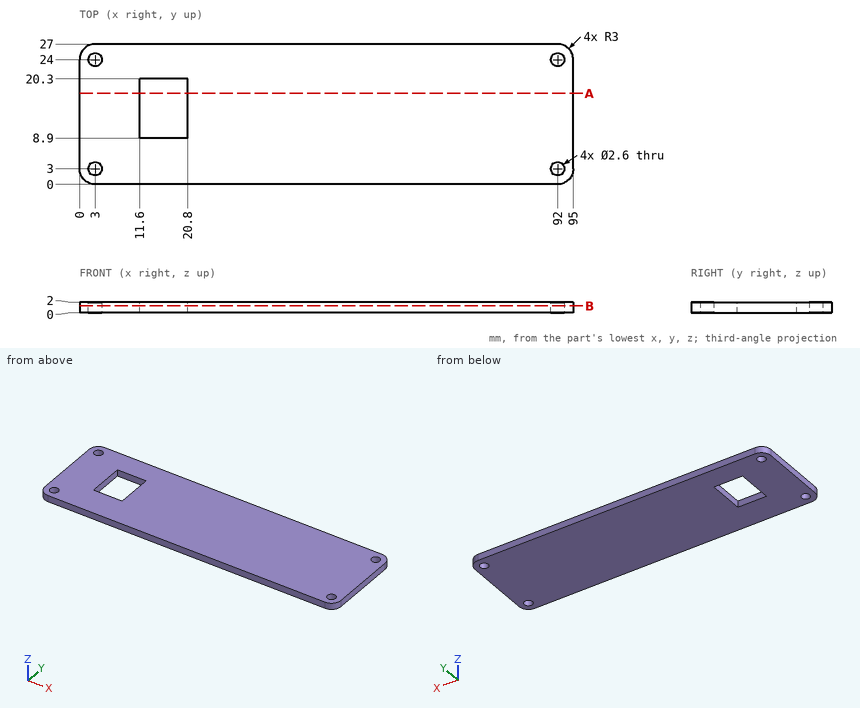
The figure shows three views and two pictorial views of one solid part (mm, origin at its lowest corner). Answer the questions. Coordinates: 2 decimals unless noted, no trailing zeros. Write each loop counter-clockwise with the first axis right and the second up, starting at its lowest first coordinate (ties: lowest second). Pieces come first, ordered by that corner, then holes. Notation, with made-up numbers: (3, 30) -> (28, 30) arc R30 cw to (28, 65) -> close; hole circle Ø9 at (53, 61). An arc over 180 degrees is marked (long way). Answer as a JSON object with one key per item and string values.
Q1. Consider line 1 (Y direction, x = 3, z = 1.15); line 2 (X direction, y = 10.75, z = 1.35); line 3 (X direction, y = 24.5, z = 1.7). Determine where each line is inside the solid, lowest interval first. Write a range as [from, to].
The answers:
{"line 1": "y = [0, 1.7], [4.3, 22.7], [25.3, 27]", "line 2": "x = [0, 11.6], [20.8, 95]", "line 3": "x = [0.04, 1.8], [4.2, 90.8], [93.2, 94.96]"}
Q2. The part is cut by section B-B on z = 1.3. Give the vertices of the cut face in (x, y), then the cut area to 3 significant figures.
The answers:
{"outline": "(0, 3) arc R3 ccw to (3, 0) -> (92, 0) arc R3 ccw to (95, 3) -> (95, 24) arc R3 ccw to (92, 27) -> (3, 27) arc R3 ccw to (0, 24) -> close; hole circle Ø2.6 at (3, 3); hole circle Ø2.6 at (3, 24); hole (11.6, 8.9) -> (20.8, 8.9) -> (20.8, 20.3) -> (11.6, 20.3) -> close; hole circle Ø2.6 at (92, 3); hole circle Ø2.6 at (92, 24)", "area": "2,430 mm2"}
Q3. The part is cut by section A-A on y = 17.5. Give the vertices of the cut face in (x, z), then the cut area to 3 significant figures.
The answers:
{"outline": "(0, 0) -> (11.6, 0) -> (11.6, 2) -> (0, 2) -> close; (20.8, 0) -> (95, 0) -> (95, 2) -> (20.8, 2) -> close", "area": "172 mm2"}
